Verification items for the finished model (mm, model axes). A direction names the side the tool comes from. Round coordinates to 2 decimals unless told otherwise and drop trailing zeros. Loops run counter-clockwise (first coordinate to the right, second up) from the corner with the lowest first, then second, coordinate; pieces in that order, holes last.
from build123d import *
from build123d.topology import SkipClean

# Parameters (mm, degrees)
SKETCH_1_R          = 3
SKETCH_1_R_2        = 1.65
EXTRUDE_1_DEPTH     = 8
EXTRUDE_START       = 0.8
SKETCH_2_R          = 4.5
SKETCH_2_R_2        = 1.65
EXTRUDE_2_DEPTH     = 0.8
SKETCH_3_R          = 2.2
CUT_EXTRUDE_1_DEPTH = 3
CHAMFER_1_SIZE      = 0.5
CHAMFER_2_SIZE      = 1
CHAMFER_2_SIZE2     = 0.577350269


with BuildPart() as part:
    # 草图1 → 凸台-拉伸1 (new body)
    with BuildSketch(Plane.XY):
        Circle(SKETCH_1_R)
        Circle(SKETCH_1_R_2, mode=Mode.SUBTRACT)
    extrude(amount=EXTRUDE_1_DEPTH)

    # 草图2 → 凸台-拉伸2 (add)
    with SkipClean():  # the faces are left unmerged after this step: merging them gives an invalid solid
        with BuildSketch(Plane(origin=(0, 0, 0), x_dir=(-1, 0, 0), z_dir=(0, 0, -1)).offset(EXTRUDE_START)):
            Circle(SKETCH_2_R)
            Circle(SKETCH_2_R_2, mode=Mode.SUBTRACT)
        extrude(amount=-EXTRUDE_2_DEPTH)

    # 草图3 → 切除-拉伸1 (cut)
    with BuildSketch(Plane(origin=(0, 0, -0.8), x_dir=(-1, 0, 0), z_dir=(0, 0, -1))):
        Circle(SKETCH_3_R)
    extrude(amount=-CUT_EXTRUDE_1_DEPTH, mode=Mode.SUBTRACT)

    # 倒角1
    chamfer_1_edges = [part.edges().sort_by_distance(p)[0] for p in [
        (4.5, 0, -0.8),
    ]]
    chamfer(chamfer_1_edges, length=CHAMFER_1_SIZE)

    # 倒角2
    chamfer_2_edges = [part.edges().sort_by_distance(p)[0] for p in [
        (-3, 0, 8),
    ]]
    chamfer_2_side = [part.faces().sort_by_distance(p)[0] for p in [
        (-3, 0, 4),
    ]]
    chamfer(chamfer_2_edges, length=CHAMFER_2_SIZE, length2=CHAMFER_2_SIZE2, reference=chamfer_2_side[0])


solid = part.part
1. Section check A-A (x = 0). Enter the section's corners in (y, z).
2. Tool access check on faces 4 (the face through (-1, -3, 0)), 5 (the face through (-2, -2, -0.8)), 6 (the face through (0, 2, 2.2)). Record the directions out of +Z, -Z, +X, -X, +Y, -Y that give a thin tool (end or side, any length) a straight path to the whole face; none if there is none.
3. Section check C-C (z = 5). Enter the section's corners in (x, y).
4. Gauge pin test, flat ends, axial feed: P1, Ø3, axis at x = 2.5, z = 3.5, coming from the +Y side; P2, Ø5, axis at x = 0, y = 0, coming from the +Z side; P3, Ø1, axis at y = 1.5, z = 2.5, coming from the +X side; P4, Ø4, axis at x = 1.5, z = 3, coming from the -Y side. Record the tip position at first contact, or that the pin passes through.
5. Section check D-D (z = 0.5). Enter the section's corners in (x, y), then the cut area to 3 significant figures.
6. Release check for a two-part mould opening along Y. For faces 1 (the face through (-2.1, 0.66, 0.68)), 2 (the face through (3.32, 3.04, -0.15)), 3 (the face through (2, -1, 8)) record: released by +Y, released by -Y, zero draft, split by the parting line, or undercut.
7. Scan lines: L1, parallel to Y at x = 0, z = 0.55; L2, parallel to Y at x = 0, z = 4; L3, parallel to Z at x = 1.5, y = 3.25. Record each from-to range of solid material in increasing order.
Taken from the geometry:
1. outline: (-4.5, -0.3) - (-4, -0.8) - (-2.2, -0.8) - (-2.2, 2.2) - (-1.65, 2.2) - (-1.65, 8) - (-2.42, 8) - (-3, 7) - (-3, 0) - (-4.5, 0) - close; (1.65, 2.2) - (2.2, 2.2) - (2.2, -0.8) - (4, -0.8) - (4.5, -0.3) - (4.5, 0) - (3, 0) - (3, 7) - (2.42, 8) - (1.65, 8) - close
2. face 4: +Z
2. face 5: -Z, +X, -X, +Y, -Y
2. face 6: -Z
3. outline: circle Ø6 at (0, 0); hole circle Ø3.3 at (0, 0)
4. P1: stops at y = 2.83
4. P2: stops at z = 8
4. P3: stops at x = 2.83
4. P4: stops at y = -3
5. outline: circle Ø6 at (0, 0); hole circle Ø4.4 at (0, 0)
5. area: 13.1 mm2
6. face 1: undercut
6. face 2: split by the parting line
6. face 3: zero draft
7. L1: y = -3 to -2.2, 2.2 to 3
7. L2: y = -3 to -1.65, 1.65 to 3
7. L3: z = -0.8 to 0
